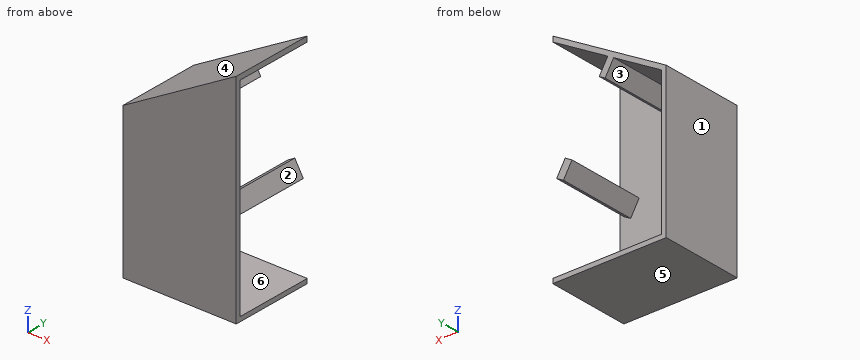
from build123d import *

# Parameters (mm, degrees)
EXTRUDE_1_DEPTH = 74
SHELL_1_T       = -4
EXTRUDE_2_DEPTH = 70


with BuildPart() as part:
    # 草图1 → 凸台-拉伸1 (new body)
    with BuildSketch(Plane(origin=(0, 0, 0), x_dir=(1, 0, 0), z_dir=(0, 1, 0))):
        Polygon((0, 0), (100, 0), (100, -190), (0, -132.264973081), align=None)
    extrude(amount=EXTRUDE_1_DEPTH)

    # 抽壳1
    shell_1_openings = [part.faces().sort_by_distance(p)[0] for p in [
        (52.985898342, 74, 81.428197876),
        (100, 37, 95),
    ]]
    offset(amount=SHELL_1_T, openings=shell_1_openings, kind=Kind.INTERSECTION)

    # 草图2 → 凸台-拉伸2 (add)
    with BuildSketch(Plane(origin=(0, 4, 0), x_dir=(1, 0, 0), z_dir=(0, 1, 0))):
        Polygon((96.535898385, -79.458149392), (89.035898385, -92.448530449), (83.035898385, -88.984428834), (90.535898385, -75.994047777), align=None)
        Polygon((51.535898385, -157.400435733), (59.035898385, -144.410054676), (53.839745962, -141.410054676), (46.339745962, -154.400435733), align=None)
    extrude(amount=EXTRUDE_2_DEPTH)


solid = part.part
Work out the finished part from the listing and answer in its coordinate system (mm). Face numbers are marked on the shaded views. A direction names the side the tool comes from. Coordinates: 2 decimals unless noted, no trailing zeros. Loops run counter-clockwise (first coordinate to the right, second up) from the corner with the lowest first, then second, coordinate; pieces in that order, holes last. Notation, with made-up numbers: (3, -30.75) -> (32, -30.75) arc R31 ccw to (32, 3.25) -> close; hole circle Ø10 at (-2.75, 18). An arc over 180 degrees is marked (long way). Write each question's results on one line, items separated by ' | '. Start each with the question number.
1) For the marked faces 1, 2 and 3, determine the directions among +Z, -Z, +X, -X, +Y, -Y from which every point of the face is accessible in a straight line to the end or side of a thin tool.
2) Flat-ended cylindrical pins translate along their axes: P1, Ø10, axis at x = 79.5, y = 39, coming from the +Z side; P2, Ø3, axis at y = 46.5, z = 77, coming from the +X side; P3, Ø3, axis at x = 51, y = 49, coming from the +Z side. Find the tip coordinate at first contact, or state that the pin passes through.
3) Find section B-B on z = 147. Determine the outline of the cut face in (x, y), then the cut area to 3 significant figures.
4) Consider line 1 along Z through (x, y) = (90, 53.5); line 2 along Z through (x, y) = (58.5, 41.5); line 3 along Y through (x, z) = (96, 73). Determine where each line is inside the solid, lowest interval first.
5) The mould has two halves that part along Z. Classify the marked faces 4, 5 and 6: pulls with the +Z half, pulls with the -Z half, needs draft (parallel to the pull), parting line crosses it, or undercut.
6) Find section C-C on x = 23. Determine the outline of the cut face in (y, z).
7) Find section D-D on z = 116.5. Determine the outline of the cut face in (x, y).
8) Find section A-A on y = 17.5. Determine the outline of the cut face in (x, z), then the cut area to 3 significant figures.
Response values:
1) face 1: +Z, -Z, -X, +Y, -Y | face 2: +X, +Y | face 3: +Y
2) P1: stops at z = 181.05 | P2: stops at x = 94.88 | P3: stops at z = 162.58
3) outline: (25.52, 0) -> (100, 0) -> (100, 4) -> (57.54, 4) -> (57.54, 74) -> (50.61, 74) -> (50.61, 4) -> (33.52, 4) -> (33.52, 74) -> (25.52, 74) -> close | area: 1,340 mm^2
4) line 1: z = 0 to 4, 76.92 to 90.78, 179.61 to 184.23 | line 2: z = 0 to 4, 144.1 to 145.34, 161.42 to 166.04 | line 3: y = 0 to 4
5) face 4: pulls with the +Z half | face 5: pulls with the -Z half | face 6: undercut
6) outline: (0, 0) -> (74, 0) -> (74, 4) -> (4, 4) -> (4, 140.93) -> (74, 140.93) -> (74, 145.54) -> (0, 145.54) -> close
7) outline: (0, 0) -> (100, 0) -> (100, 4) -> (4, 4) -> (4, 74) -> (0, 74) -> close
8) outline: (0, 0) -> (100, 0) -> (100, 4) -> (4, 4) -> (4, 129.96) -> (46.34, 154.4) -> (53.84, 141.41) -> (59.04, 144.41) -> (51.54, 157.4) -> (100, 185.38) -> (100, 190) -> (0, 132.26) -> close; (83.04, 88.98) -> (90.54, 75.99) -> (96.54, 79.46) -> (89.04, 92.45) -> close | area: 1,560 mm^2
